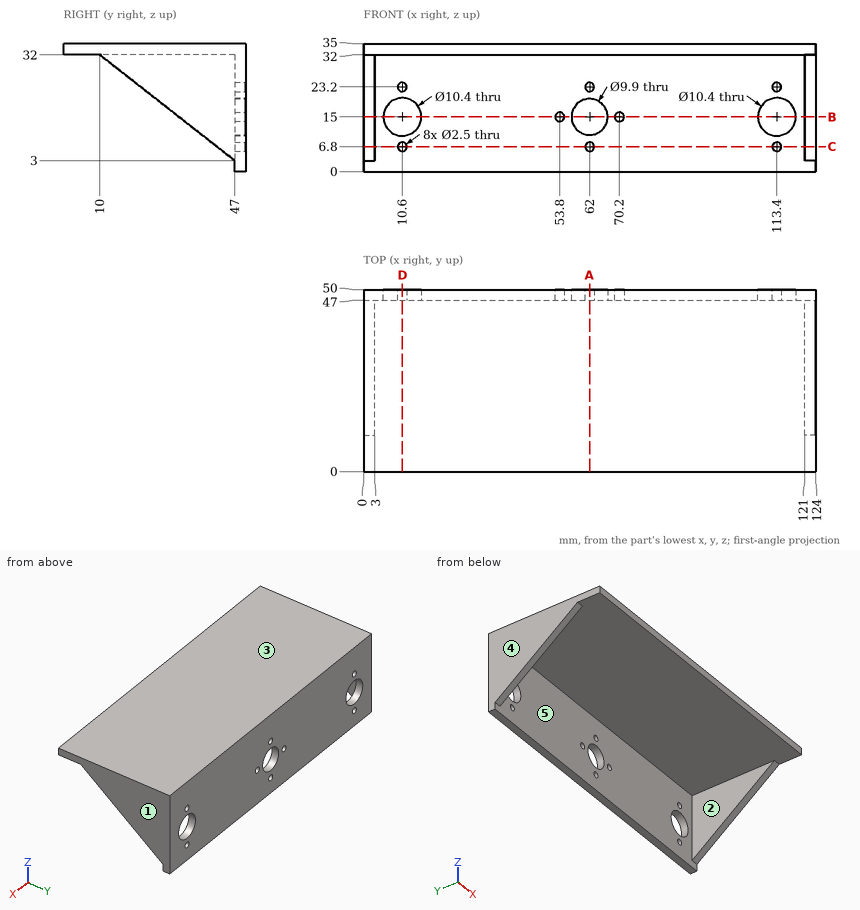
Part print with two shaded views. Sizes in mm from the minimum x, y, z corner. A direction names the side the tool comes from. Round coordinates to 2 decimals unless told otherwise and drop trailing zeros. Loops run counter-clockwise (first coordinate to the right, second up) from the corner with the lowest first, then second, coordinate; pieces in that order, holes last. Notation, with made-up numbers: (83.5, 63) - (119.5, 63) arc R8 cw to (119.5, 73) - close; hole circle Ø11 at (64.5, -40). An arc over 180 degrees is marked (long way). Answer as a JSON object with one key per item and string values.
Item 1: Tool access for the marked faces 1 and 2: list every direction of +Z, -Z, +X, -X, +Y, -Y with a clear straight run to the whole face (end or side of a thin tool).
Output:
{"face 1": "+Z, -Z, +X, +Y, -Y", "face 2": "-Z, -Y"}
Item 2: Pin check, flat tips, straight feed: pin 1 (3 mm diameter, centred on x = 10.6, z = 23.2, fed in from +Y); pin 2 (2 mm diameter, centred on x = 69, y = 13.5, fed in from -Z); pin 3 (4 mm diameter, centred on x = 70.2, z = 15, fed in from -Y). Stop position of each tip, or through.
Output:
{"pin 1": "y = 50", "pin 2": "z = 32", "pin 3": "y = 47"}
Item 3: Pull direction X, two halves, no side cores. Call the marked faces 3, 4 and 5: pulls with the +X half, pulls with the -X half, needs draft (parallel to the pull), parting line crosses it, or undercut.
Output:
{"face 3": "needs draft", "face 4": "pulls with the -X half", "face 5": "undercut"}
Item 4: Band-saw the part on D-D on x = 10.6. List the corners of the cut face in (y, z).
Output:
{"outline": "(0, 32) - (47, 32) - (47, 24.45) - (50, 24.45) - (50, 35) - (0, 35) - close; (47, 0) - (50, 0) - (50, 5.55) - (47, 5.55) - close; (47, 8.05) - (50, 8.05) - (50, 9.8) - (47, 9.8) - close; (47, 20.2) - (50, 20.2) - (50, 21.95) - (47, 21.95) - close"}
Item 5: Band-saw the part on B-B on z = 15. List the corners of the cut face in (x, y).
Output:
{"outline": "(0, 31.69) - (3, 31.69) - (3, 47) - (5.4, 47) - (5.4, 50) - (0, 50) - close; (15.8, 47) - (52.55, 47) - (52.55, 50) - (15.8, 50) - close; (55.05, 47) - (57.05, 47) - (57.05, 50) - (55.05, 50) - close; (66.95, 47) - (68.95, 47) - (68.95, 50) - (66.95, 50) - close; (71.45, 47) - (108.2, 47) - (108.2, 50) - (71.45, 50) - close; (118.6, 47) - (121, 47) - (121, 31.69) - (124, 31.69) - (124, 50) - (118.6, 50) - close"}
Item 6: Band-saw the part on C-C on z = 6.8. List the corners of the cut face in (x, y), plus the area to 3 significant figures.
Output:
{"outline": "(0, 42.15) - (3, 42.15) - (3, 47) - (9.35, 47) - (9.35, 50) - (0, 50) - close; (11.85, 47) - (60.75, 47) - (60.75, 50) - (11.85, 50) - close; (63.25, 47) - (112.15, 47) - (112.15, 50) - (63.25, 50) - close; (114.65, 47) - (121, 47) - (121, 42.15) - (124, 42.15) - (124, 50) - (114.65, 50) - close", "area": "379 mm2"}
Item 7: Band-saw the part on A-A on x = 62. List the corners of the cut face in (y, z).
Output:
{"outline": "(0, 32) - (47, 32) - (47, 24.45) - (50, 24.45) - (50, 35) - (0, 35) - close; (47, 0) - (50, 0) - (50, 5.55) - (47, 5.55) - close; (47, 8.05) - (50, 8.05) - (50, 10.05) - (47, 10.05) - close; (47, 19.95) - (50, 19.95) - (50, 21.95) - (47, 21.95) - close"}
Item 8: Wall check: L1, parallel to Z at x = 10.6, y = 48.8; L2, parallel to Z at x = 62, y = 49; L3, parallel to X at y = 49, z = 23. Give the ranges that are in metal, low to high.
Output:
{"L1": "0 to 5.55, 8.05 to 9.8, 20.2 to 21.95, 24.45 to 35", "L2": "0 to 5.55, 8.05 to 10.05, 19.95 to 21.95, 24.45 to 35", "L3": "0 to 9.37, 11.83 to 60.77, 63.23 to 112.17, 114.63 to 124"}
